Answer from the drawing. Dimensions are ordinates in mm from the lowest x, y and z of the part. A direction names the side the tool comes from. Give positions to 0.01 mm unless a question says otherwise; leave off trailing zeros. Write each loop counter-clockwise with the first axis right and the second up, starting at its lowest first coordinate (ties: lowest second). Pieces come first, ordered by that corner, then holes. Notation, with made-up numbers: (-37.5, 53) -> (-5.5, 53) arc R24 cw to (-5.5, 83) -> close; hole circle Ø8 at (5.25, 12.5). An arc over 180 degrees is marked (long way). Use a Markdown table: item, result. Add a question column.
Q1. Section D-D, the plane z = 6 is taken. Give the vertices of the cut face in (x, y) (1 decimal).
Q2. Each of these flat-tipped pins is pushed along its axis until it touches: pin 1 Ø1 at (x, z) = (5.5, 4.5) entering from -Y (1 decimal); pin 2 Ø1 at (y, z) = (4.5, 3) entering from -X; pin 3 Ø2.5 at (y, z) = (2.5, 5.5) entering from +X (1 decimal); pin 4 Ø4 at (y, z) = (3.5, 5) entering from -X. Where does it stop, or does it pass through?
Q3. Section B-B, the plane x = 1.25 is taken. Give the vertices of the cut face in (y, z).
Q4. Section A-A, the plane z = 3 is taken. State how many separate pieces and enclosed holes the cut face has, plus the area to 3 significant figures.
Q5. For a pull along Y with two mould halves and no side action, classify the marked faces 1, 2 and 3 as pulls with the +Y half, pulls with the -Y half, needs draft (parallel to the pull), parting line crosses it, or undercut.
Q6. For the marked faces 4, 5, 6 and 7, determine the directions among +Z, -Z, +X, -X, +Y, -Y from which every point of the face is accessible in a straight line to the end or side of a thin tool.
Q7. Consider line 1 (Y direction, x = 0.5, z = 1); line 2 (X direction, y = 1.25, z = 4) (1 decimal); line 3 (Z direction, x = 3.25, y = 4.5). Determine where each line is inside the solid, lowest interval first.
Q8. Section C-C, the plane y = 1.21 is taken. Give the vertices of the cut face in (x, z) (1 decimal).
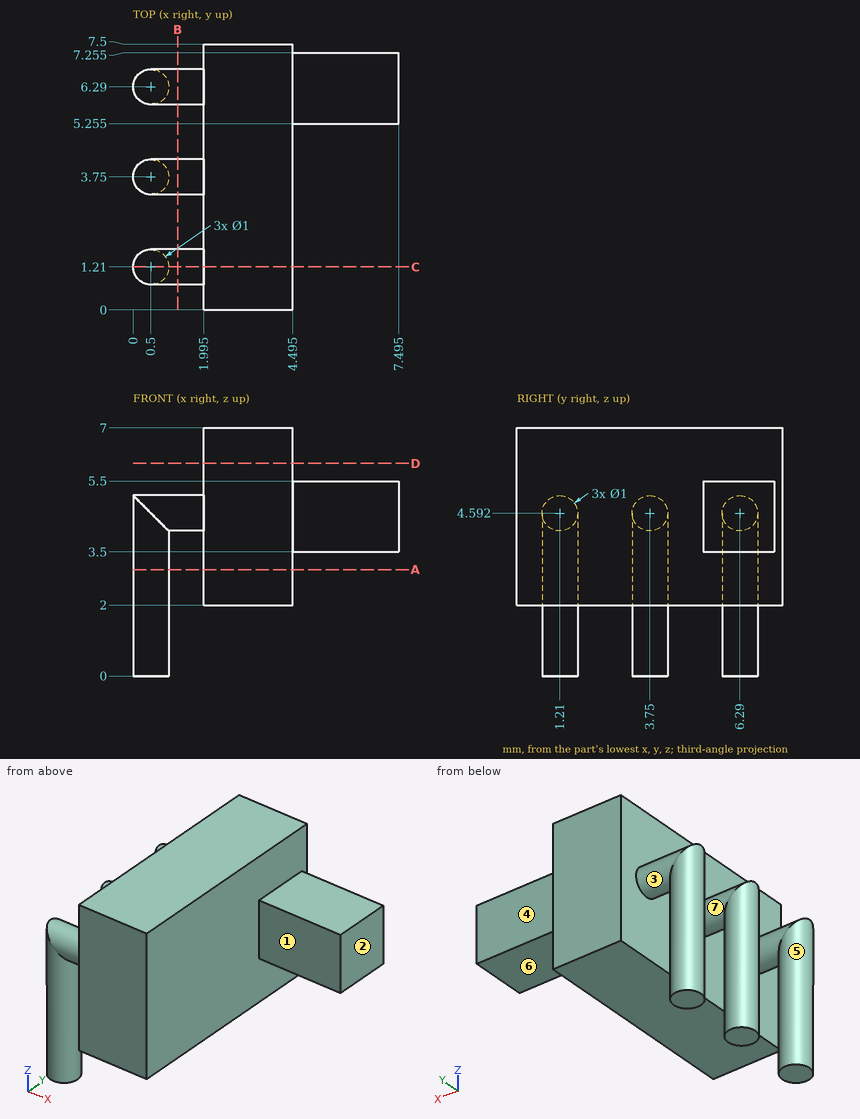
Result set:
| question | item | result |
|---|---|---|
| 1 | outline | (2, 0) -> (4.5, 0) -> (4.5, 7.5) -> (2, 7.5) -> close |
| 2 | pin 1 | stops at y = 5.3 |
| 2 | pin 2 | stops at x = 0.07 |
| 2 | pin 3 | stops at x = 4.5 |
| 2 | pin 4 | stops at x = 0 |
| 3 | outline | circle Ø1 at (1.21, 4.59); circle Ø1 at (3.75, 4.59); circle Ø1 at (6.29, 4.59) |
| 4 | separate pieces | 4 |
| 4 | enclosed holes | 0 |
| 4 | area | 21.1 mm2 |
| 5 | face 1 | pulls with the -Y half |
| 5 | face 2 | needs draft |
| 5 | face 3 | undercut |
| 6 | face 4 | +Z, -Z, +X, +Y |
| 6 | face 5 | -Z |
| 6 | face 6 | -Z, +X, +Y, -Y |
| 6 | face 7 | none |
| 7 | line 1 | y = 0.71 to 1.71, 3.25 to 4.25, 5.79 to 6.79 |
| 7 | line 2 | x = 0 to 1, 2 to 4.5 |
| 7 | line 3 | z = 2 to 7 |
| 8 | outline | (0, 0) -> (1, 0) -> (1, 4.1) -> (2, 4.1) -> (2, 2) -> (4.5, 2) -> (4.5, 7) -> (2, 7) -> (2, 5.1) -> (0, 5.1) -> close |
